CAD build for the part. Positions are in the model's coordinates, mm. A direction names the side the tool comes from. Coordinates: 2 decimals unless noted, no trailing zeros. Write each loop counter-clockwise with the first axis right and the second up, starting at its lowest first coordinate (ties: lowest second). Pieces come first, ordered by that corner, then holes. Notation, with made-up numbers: (62, 0) - (84, 0) arc R29 ccw to (84, 26) - close; hole circle Ø8 at (83, -18.75). An arc over 180 degrees is marked (long way). Answer in a Markdown table with one row per item. Add a question column.
Q1. Band-saw the part on B-B (x = 15). List the corners of the cut face in (y, z), and give its area (3 significant figures).
Q2. Two-plate mould, pull along Z, no slides. Class faces 1 (the flat face through (7.16, 14.23, -1.48)), 2 (the flat face through (3.6, 6.4, 11)), 3 (the flat face through (0, 10, 5)): +Z half, -Z half, draft (parallel to the pull), parting line (faces both ways), or undercut.
Q3. Band-saw the part on C-C (z = -0.75). List the corners of the cut face in (x, y).
Q4. Band-saw the part on D-D (z = 1.5). List the corners of the cut face in (x, y), and give its area (3 significant figures).
Q5. 3-axis set-ups, long thin cutter, end or side, ignore diameter. For faces 4 (the flat face through (21.592, 17, -1)), 5 (the flat face through (20, -1, 6)), 6 (the flat face through (5, 3, 10)), 7 (the flat face through (12.1, 4, 10.5)), 8 (the flat face through (-1, 20, 7)): which of +Z, -Z, +X, -X, +Y, -Y reach the whole face in a straight line?
Q6. Band-saw the part on A-A (y = 14). List the corners of the cut face in (x, z).
Q7. Drill centre lines: line 1 along Z through (x, y) = (18.5, 1); line 2 along Y through (x, z) = (9, 2.5). Where is each one in solid material? Low to high. Write a range as from..to.
Q8. Pin check, flat tips, straight feed: pin 1 (4 mm diameter, centred on x = 9, y = 16.5, fed in from +Z); pin 2 (3 mm diameter, centred on x = 2.5, z = 3, fed in from +Y); pin 3 (2 mm diameter, centred on y = 0.5, z = 6, fed in from +X); pin 4 (6 mm diameter, centred on y = 24, z = 4, fed in from +X). Stop position of each tip, or through.
```python
from build123d import *

# Parameters (mm, degrees)
F2_DEPTH  = 7
F4_DEPTH  = 3
F5_DEPTH  = 7
F7_DEPTH  = 1.5
F8_R      = 0.99999
F10_DEPTH = 1


# Not quite as in the source:
# - a fillet or chamfer is up to 0.001 mm smaller than in the source, because OpenCascade refuses the exact size


with BuildPart() as f2:
    # F1 (on offset) → F2 (new body)
    with BuildSketch(Plane.XY.offset(4)):
        Polygon((20, 0), (0, 0), (0, 20), (-2.5, 20), (-2.5, -2.5), (20, -2.5), align=None)
    extrude(amount=F2_DEPTH)



with BuildPart() as f4:
    # F3 (on Top) → F4 (new body)
    with BuildSketch(Plane.XY):
        Polygon((21.591883092, 18.7634559673), (21.591883092, 14.5208152802), (4.5710678119, -2.5), (8.75, -2.5), (20, -2.5), (27.9713179916, 16.5624991059), (22.2989825486, 22.2989889792), (16.5624926754, 27.9713244222), (-2.5, 20), (-2.5, 8.75), (-2.5, 4.5710678119), (14.5208152802, 21.591883092), (18.7634559673, 21.591883092), (20.1776695297, 20.1776695297), align=None)
    extrude(amount=-F4_DEPTH)


with BuildPart() as f2_1:
    add(f2.part)

    add(f4.part)  # F5 merges F4
    # F1 (on offset) → F5 (join)
    with BuildSketch(Plane.XY.offset(4)):
        Polygon((20, 0), (0, 0), (0, 20), (-2.5, 20), (-2.5, -2.5), (20, -2.5), align=None)
    extrude(amount=-F5_DEPTH)

    # F6 (on face) → F7 (join)
    with BuildSketch(Plane(origin=(20.1776695297, 20.1776695297, 0), x_dir=(0.7071067812, -0.7071067812, 0), z_dir=(-0.7071067812, -0.7071067812, 0))):
        with BuildLine():
            Line((-1, -3), (1, -3))
            ThreePointArc((1, -3), (0, -2), (-1, -3))
        make_face()
    extrude(amount=F7_DEPTH)

    # F8 (radius 1 in the source; OpenCascade refuses exactly that, so slightly less here)
    f8_edges = [f2_1.edges().sort_by_distance(p)[0] for p in [
        (19.117009, 19.117009, -2),
    ]]
    fillet(f8_edges, radius=F8_R)

    # F9 (on face) → F10 (join)
    with BuildSketch(Plane.XY.offset(11)):
        Polygon((4, 20), (-2.5, 20), (-2.5, -2.5), (20, -2.5), (20, 4), (4, 4), align=None)
    extrude(amount=-F10_DEPTH)


solid = f2_1.part
```
Checked values:
| question | item | result |
|---|---|---|
| 1 | outline | (-2.5, -3) - (7.93, -3) - (7.93, 0) - (0, 0) - (0, 10) - (4, 10) - (4, 11) - (-2.5, 11) - close; (21.59, -3) - (27.32, -3) - (27.32, 0) - (21.59, 0) - close |
| 1 | area | 80.0 mm² |
| 2 | face 1 | draft |
| 2 | face 2 | +Z half |
| 2 | face 3 | undercut |
| 3 | outline | (-2.5, -2.5) - (20, -2.5) - (27.97, 16.56) - (22.3, 22.3) - (16.56, 27.97) - (-2.5, 20) - close; hole (0, 0) - (7.07, 0) - (21.59, 14.52) - (21.59, 18.76) - (18.76, 21.59) - (14.52, 21.59) - (0, 7.07) - close |
| 4 | outline | (-2.5, -2.5) - (20, -2.5) - (20, 0) - (0, 0) - (0, 20) - (-2.5, 20) - close |
| 4 | area | 106 mm² |
| 5 | face 4 | +Z, -Z |
| 5 | face 5 | +Z, +X, +Y, -Y |
| 5 | face 6 | +X, +Y |
| 5 | face 7 | +Z, +X, +Y |
| 5 | face 8 | +Z, +X, -X, +Y |
| 6 | outline | (-2.5, -3) - (6.93, -3) - (6.93, 0) - (0, 0) - (0, 10) - (4, 10) - (4, 11) - (-2.5, 11) - close; (21.07, -3) - (26.9, -3) - (26.9, 0) - (21.07, 0) - close |
| 7 | line 1 | z = -3..0, 10..11 |
| 7 | line 2 | y = -2.5..0 |
| 8 | pin 1 | stops at z = 0 |
| 8 | pin 2 | stops at y = 0 |
| 8 | pin 3 | stops at x = 20 |
| 8 | pin 4 | passes through |
